Part model, mm, in its own coordinate system. Face numbers are marked on the shaded views. A direction names the side the tool comes from. Round coordinates to 2 decimals unless told otherwise and drop trailing zeros. Order: outer loops, then holes, each group sorted by start corner. A loop starts at its lowest first (then second) coordinate and runs counter-clockwise, first axis right, second up. Notation, with made-up numbers: (11, 1) - (53, 1) arc R25 ccw to (53, 27) - close; hole circle Ø6 at (-18.5, 66). An arc over 180 degrees is marked (long way). Answer as a JSON object with one key per item and string values.
```python
from build123d import *

# Parameters (mm, degrees)
SALIENTE_EXTRUIR1_DEPTH  = 42.3
CROQUIS3_W               = 40.9
CROQUIS3_H               = 56.9
CORTAR_EXTRUIR1_DEPTH    = 1.3
CROQUIS5_W               = 42.3
CROQUIS5_H               = 2.8
CORTAR_EXTRUIR2_DEPTH    = 7.8
CROQUIS6_W               = 40.9
CROQUIS6_H               = 26.5
CORTAR_EXTRUIR3_DEPTH    = 1.3
CROQUIS8_W               = 39.7
CROQUIS8_H               = 56.9
CORTAR_EXTRUIR4_DEPTH    = 6.5
CROQUIS9_W               = 39.7
CROQUIS9_H               = 32.2
CORTAR_EXTRUIR5_DEPTH    = 7.3
CROQUIS10_W              = 21.7
CROQUIS10_H              = 50.979199381
CROQUIS10_W_2            = 19.3
CROQUIS10_H_2            = 48.579199381
SALIENTE_EXTRUIR2_DEPTH  = 6.5
REDONDEO6_R              = 1
REDONDEO7_R              = 1
CROQUIS17_W              = 39.7
CROQUIS17_H              = 32.2
SALIENTE_EXTRUIR4_DEPTH  = 6
SALIENTE_EXTRUIR5_DEPTH  = 1.3
CORTAR_EXTRUIR6_DEPTH    = 21
REDONDEO8_R              = 2
REDONDEO10_R             = 2
CROQUIS26_R              = 7.1
CROQUIS26_R_2            = 4.35
SALIENTE_EXTRUIR7_DEPTH  = 6.5
CORTAR_EXTRUIR7_START    = -44
CROQUIS27_R              = 4.35
CORTAR_EXTRUIR7_DEPTH    = 44
CROQUIS28_W              = 19.3
CROQUIS28_H              = 2
SALIENTE_EXTRUIR8_DEPTH  = 6.5
REDONDEO11_R             = 2
REDONDEO12_R             = 2
CROQUIS30_R              = 4.75
CROQUIS30_R_2            = 1.25
SALIENTE_EXTRUIR9_DEPTH  = 6.5
CROQUIS33_W              = 19.3
CROQUIS33_H              = 2.5
SALIENTE_EXTRUIR11_DEPTH = 6.5
CORTAR_EXTRUIR8_DEPTH    = 4.1
CROQUIS23_W              = 4
CROQUIS23_H              = 4
SALIENTE_EXTRUIR12_DEPTH = 3.7
NERVIO5_REACH            = 61.555
CROQUIS39_WALL_W         = 124.026264302
CROQUIS39_WALL_H         = 52.8
NERVIO7_REACH            = 61.555
CROQUIS43_WALL_W         = 124.026264302
CROQUIS43_WALL_H         = 52.8
CROQUIS44_W              = 42.3
CROQUIS44_H              = 3
SALIENTE_EXTRUIR13_DEPTH = 4.7
REDONDEO13_R             = 2
REDONDEO14_R             = 2


with BuildPart() as part:
    # Croquis1 → Saliente-Extruir1 (new body)
    with BuildSketch(Plane(origin=(0, 0, 0), x_dir=(0, 0, -1), z_dir=(1, 0, 0))):
        Polygon((-38.13826087, -2.227336957), (21.56173913, -2.227336957), (21.56173913, 23.672663043), (29.76173913, 23.672663043), (29.76173913, -2.261684783), (29.76173913, -11.327336957), (-38.13826087, -11.327336957), align=None)
    extrude(amount=-SALIENTE_EXTRUIR1_DEPTH)

    # Croquis3 → Cortar-Extruir1 (cut)
    with BuildSketch(Plane(origin=(0, -2.227336957, 0), x_dir=(1, 0, 0), z_dir=(0, 1, 0))):
        with Locations((-21.15, -6.88826087)):
            Rectangle(CROQUIS3_W, CROQUIS3_H)
    extrude(amount=-CORTAR_EXTRUIR1_DEPTH, mode=Mode.SUBTRACT)

    # Croquis5 → Cortar-Extruir2 (cut)
    with BuildSketch(Plane(origin=(0, -2.227336957, 0), x_dir=(1, 0, 0), z_dir=(0, 1, 0))):
        with Locations((-21.15, -36.73826087)):
            Rectangle(CROQUIS5_W, CROQUIS5_H)
    extrude(amount=-CORTAR_EXTRUIR2_DEPTH, mode=Mode.SUBTRACT)

    # Croquis6 → Cortar-Extruir3 (cut)
    with BuildSketch(Plane.XY.offset(-21.56173913)):
        with Locations((-21.15, 9.722663043)):
            Rectangle(CROQUIS6_W, CROQUIS6_H)
    extrude(amount=-CORTAR_EXTRUIR3_DEPTH, mode=Mode.SUBTRACT)

    # Croquis8 → Cortar-Extruir4 (cut)
    with BuildSketch(Plane(origin=(0, -3.527336957, 0), x_dir=(1, 0, 0), z_dir=(0, 1, 0))):
        with Locations((-21.15, -6.88826087)):
            Rectangle(CROQUIS8_W, CROQUIS8_H)
    extrude(amount=-CORTAR_EXTRUIR4_DEPTH, mode=Mode.SUBTRACT)

    # Croquis9 → Cortar-Extruir5 (cut)
    with BuildSketch(Plane.XY.offset(-21.56173913)):
        with Locations((-21.15, 6.072663043)):
            Rectangle(CROQUIS9_W, CROQUIS9_H)
    extrude(amount=-CORTAR_EXTRUIR5_DEPTH, mode=Mode.SUBTRACT)

    # Croquis10 → Saliente-Extruir2 (add)
    with BuildSketch(Plane(origin=(0, -10.027336957, 0), x_dir=(1, 0, 0), z_dir=(0, 1, 0))):
        with Locations((-21.15, -5.42786056)):
            Rectangle(CROQUIS10_W, CROQUIS10_H)
        with Locations((-21.15, -5.427860561)):
            Rectangle(CROQUIS10_W_2, CROQUIS10_H_2, mode=Mode.SUBTRACT)
    extrude(amount=SALIENTE_EXTRUIR2_DEPTH)

    # Redondeo6
    redondeo6_edges = [part.edges().sort_by_distance(p)[0] for p in [
        (-30.8, -6.777336957, -18.86173913),
        (-11.5, -6.777336957, -18.86173913),
        (-11.5, -6.777336957, 29.717460251),
        (-30.8, -6.777336957, 29.717460251),
    ]]
    fillet(redondeo6_edges, radius=REDONDEO6_R)

    # Redondeo7
    redondeo7_edges = [part.edges().sort_by_distance(p)[0] for p in [
        (-10.3, -6.777336957, -20.06173913),
        (-10.3, -6.777336957, 30.917460251),
        (-32, -6.777336957, 30.917460251),
        (-32, -6.777336957, -20.06173913),
    ]]
    fillet(redondeo7_edges, radius=REDONDEO7_R)

    # Croquis17 → Saliente-Extruir4 (add)
    with BuildSketch(Plane.XY.offset(-28.86173913)):
        with Locations((-21.15, 6.072663043)):
            Rectangle(CROQUIS17_W, CROQUIS17_H)
    extrude(amount=SALIENTE_EXTRUIR4_DEPTH)

    # Croquis18 → Saliente-Extruir5 (add)
    with BuildSketch(Plane.XY.offset(-22.86173913)):
        Polygon((-41.6, 22.972663043), (-41.6, -3.527336957), (-41, -3.527336957), (-41, -10.027336957), (-1.3, -10.027336957), (-1.3, -3.527336957), (-0.7, -3.527336957), (-0.7, 22.972663043), align=None)
    extrude(amount=SALIENTE_EXTRUIR5_DEPTH)

    # Croquis19 → Cortar-Extruir6 (cut)
    with BuildSketch(Plane(origin=(0, 23.672663043, 0), x_dir=(1, 0, 0), z_dir=(0, 1, 0))):
        with BuildLine():
            Line((-42.3, 23.48173913), (-42.3, 21.56173913))
            Line((-42.3, 21.56173913), (0, 21.56173913))
            Line((0, 21.56173913), (0, 23.48173913))
            ThreePointArc((0, 23.48173913), (-21.15, 24.415477395), (-42.3, 23.48173913))
        make_face()
    extrude(amount=-CORTAR_EXTRUIR6_DEPTH, mode=Mode.SUBTRACT)

    # Redondeo8
    redondeo8_edges = [part.edges().sort_by_distance(p)[0] for p in [
        (-42.3, 6.172663043, -29.76173913),
        (-21.15, 23.672663043, -29.76173913),
        (-21.15, -11.327336957, -29.76173913),
        (0, 6.172663043, -29.76173913),
    ]]
    fillet(redondeo8_edges, radius=REDONDEO8_R)

    # Redondeo10
    # the kernel refuses this fillet: 2 mm, written as the material it takes off along each edge
    with BuildSketch(Plane(origin=(-40.3, -9.327336957, -27.76173913), x_dir=(-1, 0, 0), z_dir=(0, -1, 0))) as redondeo10_piece_1_section:
        Polygon((0, 0), (REDONDEO10_R, 0), (REDONDEO10_R, REDONDEO10_R), (0, REDONDEO10_R), align=None)
    redondeo10_piece_1 = extrude(amount=REDONDEO10_R, mode=Mode.PRIVATE)
    redondeo10_piece_1 = redondeo10_piece_1 - Plane(origin=(-40.3, -9.327336957, -27.76173913), x_dir=(0.7071067811865475, 0, 0.7071067811865475), z_dir=(0, -1, 0)) * Sphere(REDONDEO10_R, mode=Mode.PRIVATE)
    add(redondeo10_piece_1, mode=Mode.SUBTRACT)
    with BuildSketch(Plane(origin=(-2, -9.327336957, -27.76173913), x_dir=(0, -1, 0), z_dir=(1, 0, 0))) as redondeo10_piece_2_section:
        Polygon((0, 0), (REDONDEO10_R, 0), (REDONDEO10_R, REDONDEO10_R), (0, REDONDEO10_R), align=None)
    redondeo10_piece_2 = extrude(amount=REDONDEO10_R, mode=Mode.PRIVATE)
    redondeo10_piece_2 = redondeo10_piece_2 - Plane(origin=(-2, -9.327336957, -27.76173913), x_dir=(0, 0.7071067811865475, 0.7071067811865475), z_dir=(1, 0, 0)) * Sphere(REDONDEO10_R, mode=Mode.PRIVATE)
    add(redondeo10_piece_2, mode=Mode.SUBTRACT)
    with BuildSketch(Plane(origin=(-42.3, -11.327336957, -27.76173913), x_dir=(1, 0, 0), z_dir=(0, 0, 1)), Plane(origin=(0, -11.327336957, -27.76173913), x_dir=(0, 1, 0), z_dir=(0, 0, 1))) as redondeo10_piece_3:
        with BuildLine():
            CenterArc((REDONDEO10_R, REDONDEO10_R), REDONDEO10_R, 180, 90)
            Line((0, REDONDEO10_R), (0, 0))
            Line((0, 0), (REDONDEO10_R, 0))
        make_face()
    extrude(amount=70.9, mode=Mode.SUBTRACT)

    # Croquis26 → Saliente-Extruir7 (add)
    with BuildSketch(Plane(origin=(0, -10.027336957, 0), x_dir=(1, 0, 0), z_dir=(0, 1, 0))):
        with Locations(Location((-21.15, -5.18826087, 0), (0, 0, 90))):
            Circle(CROQUIS26_R)
        with Locations(Location((-21.15, -5.18826087, 0), (0, 0, 270))):
            Circle(CROQUIS26_R_2, mode=Mode.SUBTRACT)
    extrude(amount=SALIENTE_EXTRUIR7_DEPTH)

    # Croquis27 → Cortar-Extruir7 (cut)
    with BuildSketch(Plane(origin=(0, -10.027336957, 0), x_dir=(1, 0, 0), z_dir=(0, 1, 0)).offset(CORTAR_EXTRUIR7_START)):
        with Locations(Location((-21.15, -5.18826087, 0), (0, 0, 90))):
            Circle(CROQUIS27_R)
    extrude(amount=CORTAR_EXTRUIR7_DEPTH, mode=Mode.SUBTRACT)

    # Croquis28 → Saliente-Extruir8 (add)
    with BuildSketch(Plane(origin=(0, -10.027336957, 0), x_dir=(1, 0, 0), z_dir=(0, 1, 0))):
        with Locations((-21.15, 1.769114844)):
            Rectangle(CROQUIS28_W, CROQUIS28_H)
        with Locations((-21.15, -12.145636583)):
            Rectangle(CROQUIS28_W, CROQUIS28_H)
    extrude(amount=SALIENTE_EXTRUIR8_DEPTH)

    # Redondeo11
    redondeo11_edges = [part.edges().sort_by_distance(p)[0] for p in [
        (-30.8, -6.777336957, -0.769114844),
        (-11.5, -6.777336957, -0.769114844),
        (-11.5, -6.777336957, 11.145636583),
        (-30.8, -6.777336957, 11.145636583),
    ]]
    fillet(redondeo11_edges, radius=REDONDEO11_R)

    # Redondeo12
    redondeo12_edges = [part.edges().sort_by_distance(p)[0] for p in [
        (-30.8, -6.777336957, -2.769114844),
        (-11.5, -6.777336957, -2.769114844),
        (-30.8, -6.777336957, 13.145636583),
        (-11.5, -6.777336957, 13.145636583),
    ]]
    fillet(redondeo12_edges, radius=REDONDEO12_R)

    # Croquis30 → Saliente-Extruir9 (add)
    # profile 1 of 2: a face of its own
    with BuildSketch(Plane(origin=(0, -10.027336957, 0), x_dir=(1, 0, 0), z_dir=(0, 1, 0))):
        with Locations(Location((-21.15, 11.315426987, 0), (0, 0, 90))):
            Circle(CROQUIS30_R)
        with Locations(Location((-21.15, 11.315426987, 0), (0, 0, 270))):
            Circle(CROQUIS30_R_2, mode=Mode.SUBTRACT)
    # profile 2 of 2: a face of its own
    with BuildSketch(Plane(origin=(0, -10.027336957, 0), x_dir=(1, 0, 0), z_dir=(0, 1, 0))):
        with Locations(Location((-21.15, -21.691948726, 0), (0, 0, 90))):
            Circle(CROQUIS30_R)
        with Locations(Location((-21.15, -21.691948726, 0), (0, 0, 90))):
            Circle(CROQUIS30_R_2, mode=Mode.SUBTRACT)
    extrude(amount=SALIENTE_EXTRUIR9_DEPTH)

    # Croquis33 → Saliente-Extruir11 (add)
    with BuildSketch(Plane(origin=(0, -10.027336957, 0), x_dir=(1, 0, 0), z_dir=(0, 1, 0))):
        with Locations((-21.15, 16.519944868)):
            Rectangle(CROQUIS33_W, CROQUIS33_H)
        with Locations((-21.15, 6.110909106)):
            Rectangle(CROQUIS33_W, CROQUIS33_H)
        with Locations((-21.15, -16.487430845)):
            Rectangle(CROQUIS33_W, CROQUIS33_H)
        with Locations((-21.15, -26.896466607)):
            Rectangle(CROQUIS33_W, CROQUIS33_H)
    extrude(amount=SALIENTE_EXTRUIR11_DEPTH)

    # Croquis34 → Cortar-Extruir8 (cut)
    with BuildSketch(Plane.XY.offset(35.33826087)):
        Polygon((-1.3, -10.027336957), (-1.3, -3.527336957), (-0.7, -3.527336957), (-0.7, -2.227336957), (0, -2.227336957), (0, -10.027336957), align=None)
        Polygon((-42.3, -2.227336957), (-42.3, -10.027336957), (-41, -10.027336957), (-41, -3.527336957), (-41.6, -3.527336957), (-41.6, -2.227336957), align=None)
    extrude(amount=-CORTAR_EXTRUIR8_DEPTH, mode=Mode.SUBTRACT)

    # Croquis23 → Saliente-Extruir12 (add)
    with BuildSketch(Plane(origin=(0, -10.027336957, 0), x_dir=(1, 0, 0), z_dir=(0, 1, 0))):
        with Locations((-6.76, -25.93826087)):
            Rectangle(CROQUIS23_W, CROQUIS23_H)
        with Locations((-35.54, -25.93826087)):
            Rectangle(CROQUIS23_W, CROQUIS23_H)
    extrude(amount=SALIENTE_EXTRUIR12_DEPTH)

    # Croquis39 wall → Nervio5 (add, up to next)
    with BuildSketch(Plane(origin=(-40.25, -8.777336957, 4.83826087), x_dir=(0.514495755428, -0.857492925713, 0), z_dir=(0.857492925713, 0.514495755428, 0)), mode=Mode.PRIVATE) as nervio5_sk1:
        Rectangle(CROQUIS39_WALL_W, CROQUIS39_WALL_H)
    nervio5_tool1 = extrude(nervio5_sk1.sketch, amount=-NERVIO5_REACH, mode=Mode.PRIVATE) - part.part
    add(nervio5_tool1.solids().sort_by_distance((-40.25, -8.777336957, 4.83826087))[0])

    # Croquis43 wall → Nervio7 (add, up to next)
    with BuildSketch(Plane(origin=(-2.05, -8.777336957, 4.83826087), x_dir=(-0.514495755428, -0.857492925713, 0), z_dir=(0.857492925713, -0.514495755428, 0)), mode=Mode.PRIVATE) as nervio7_sk1:
        Rectangle(CROQUIS43_WALL_W, CROQUIS43_WALL_H)
    nervio7_tool1 = extrude(nervio7_sk1.sketch, amount=NERVIO7_REACH, mode=Mode.PRIVATE) - part.part
    add(nervio7_tool1.solids().sort_by_distance((-2.05, -8.777336957, 4.83826087))[0])

    # Croquis44 → Saliente-Extruir13 (add)
    with BuildSketch(Plane.XY.offset(-21.56173913)):
        with Locations((-21.15, 22.172663043)):
            Rectangle(CROQUIS44_W, CROQUIS44_H)
    extrude(amount=-SALIENTE_EXTRUIR13_DEPTH)

    # Redondeo13
    redondeo13_edges = [part.edges().sort_by_distance(p)[0] for p in [
        (-21.15, 2.672663043, -24.415477395),
        (-21.15, 20.672663043, -24.415477395),
    ]]
    fillet(redondeo13_edges, radius=REDONDEO13_R)

    # Redondeo14
    redondeo14_edges = [part.edges().sort_by_distance(p)[0] for p in [
        (-21.15, 23.672663043, -21.56173913),
    ]]
    fillet(redondeo14_edges, radius=REDONDEO14_R)


solid = part.part
```
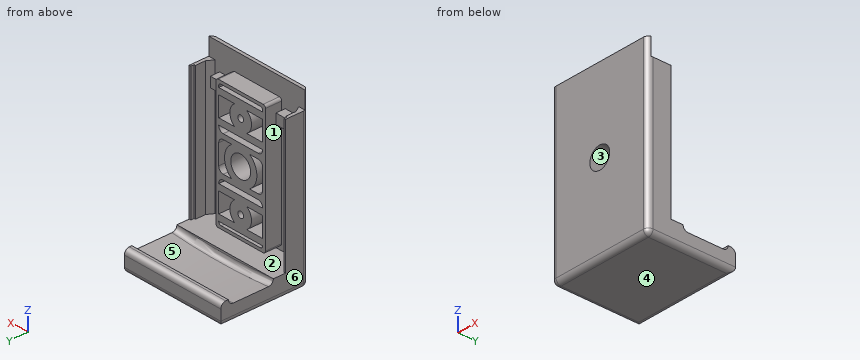
Item 1: Two-plate mould, pull along X, no slides. Class the marked faces 4, 5 and 6: pulls with the +X half, pulls with the -X half, needs draft (parallel to the pull), parting line crosses it, or undercut.
Taken from the geometry:
{"face 4": "needs draft", "face 5": "undercut", "face 6": "pulls with the -X half"}
Item 2: Tool access for the marked faces 1, 2 and 3: list every direction of +Z, -Z, +X, -X, +Y, -Y with a clear straight run to the whole face (end or side of a thin tool).
Taken from the geometry:
{"face 1": "+Z, +Y", "face 2": "+Y", "face 3": "+Y, -Y"}
Item 3: Cut at B-B (z = -6.5). Write the cut outline in (x, y).
Taken from the geometry:
{"outline": "(-42.3, -9.33) arc R2 ccw to (-40.3, -11.33) - (-2, -11.33) arc R2 ccw to (0, -9.33) - (0, -2.23) - (-0.7, -2.23) - (-0.7, -3.53) - (-1.3, -3.53) - (-1.3, -7.53) - (-2.8, -10.03) - (-10.3, -10.03) - (-10.3, -3.53) - (-32, -3.53) - (-32, -10.03) - (-39.5, -10.03) - (-41, -7.53) - (-41, -3.53) - (-41.6, -3.53) - (-41.6, -2.23) - (-42.3, -2.23) - close"}
Item 4: Cut at C-C (y = 7.5). Write the cut outline in (x, z).
Taken from the geometry:
{"outline": "(-42.3, -27.76) arc R2 ccw to (-40.3, -29.76) - (-2, -29.76) arc R2 ccw to (0, -27.76) - (0, -23.48) arc R240 cw to (-42.3, -23.48) - close"}
Item 5: Drop flat-ended pins along their axis: P1, Ø1.1, axis at x = -7.5, y = -7.5, coming from the +Z side; P2, Ø4, axis at x = -15, y = 10, coming from the +Z side; P3, Ø6.5, axis at x = -14, z = 5, coming from the +Y side. Give the stop position or say it passes through.
Taken from the geometry:
{"P1": "z = 27.94", "P2": "z = -24.28", "P3": "y = -3.53"}
Item 6: Cut at A-A (y = -4.5). State how many separate pieces and enclosed holes the cut face has, plus the area to 3 significant figures.
Taken from the geometry:
{"separate pieces": "2", "enclosed holes": "13", "area": "1,140 mm2"}
Item 7: Probe L1, parallel to Z at x = -7, y = -7.5; L2, parallel to X at y = -8, z = -15; L3, parallel to Y at x = -15, z = -10. List the from-to ranges inside material, lowest first. Write a range as from..to.
Taken from the geometry:
{"L1": "-29.76..-21.56, 23.94..27.94", "L2": "-42.3..-40.72, -32..-30.8, -24.15..-18.15, -11.5..-10.3, -1.58..0", "L3": "-11.33..-10.03"}
